Geometry: final body of the model. Coordinates: model frame, mm. Face numbers are marked on the shaded views. A direction names the side the tool comes from. Give positions to 0.01 mm unless a question says otherwise; leave off trailing zeros. Write each loop counter-clockwise with the first axis right and the second up, starting at its lowest first coordinate (ties: lowest second). Pieces come first, ordered by that corner, then holes. Notation, with made-up numbers: (27, 10.5) -> (82, 10.5) arc R18 ccw to (82, 26.5) -> close; hole circle Ø4 at (-2, 69.5). An arc over 180 degrees is marked (long way). Answer as a JSON object with one key per item and string values. Group by question number.
(1) Section query C-C on y = 12. Output: boundary loops of the cut face in (x, z).
(2) Contact query for flat-ended pins moving along their axis: pin 1 Ø4.5 at (x, y) = (6.46, 12) entering from -Z; pin 2 Ø6 at (x, z) = (-3, -2) entering from -Y; pin 3 Ø3 at (x, z) = (-11, -11) entering from +Y. Output: stop coordinate, or through.
(3) Material intervals for probe 1 along X at (y, z) = (1.95, 0); probe 2 along Z at (x, y) = (11, 8.25); probe 3 along Y at (x, z) = (10.5, -2.5), sorted ascending.
(4) Set-up query: the marked faces 1 and 2. Return all of +Z, -Z, +X, -X, +Y, -Y with unobstructed straight access to the full face (end or side cutting, diameter ignored); none if empty.
(5) Section query A-A on x = 0. Output: boundary loops of the cut face in (y, z), plus the area to 3 significant figures.
(6) Section query B-B on z = -6.25. Output: boundary loops of the cut face in (x, y), plus the area to 3 significant figures.
(7) Section query D-D on y = 9.25. Output: boundary loops of the cut face in (x, z), plus the area to 3 significant figures.
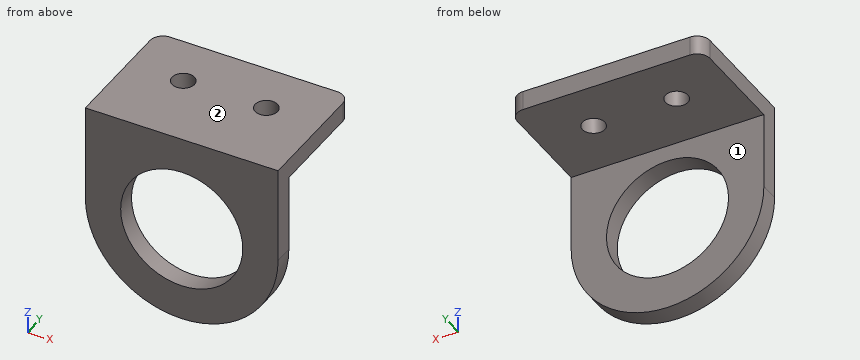
from build123d import *

# Parameters (mm, degrees)
SKETCH_1_R          = 9.5
EXTRUDE_2_DEPTH     = 3
SKETCH_9_W          = 30
SKETCH_9_H          = 20
EXTRUDE_3_DEPTH     = 3
SKETCH_10_R         = 1.75
CUT_EXTRUDE_1_DEPTH = 37.796738986
FILLET_6_R          = 2


with BuildPart() as part:
    # 草图1 → 凸台-拉伸2 (new body)
    with BuildSketch(Plane(origin=(0, 0, 0), x_dir=(1, 0, 0), z_dir=(0, 1, 0))):
        with BuildLine():
            Line((15, -15), (15, 0))
            ThreePointArc((15, 0), (0, 15), (-15, 0))
            Line((-15, 0), (-15, -15))
            Line((-15, -15), (15, -15))
        make_face()
        with Locations(Location((0, 0, 0), (0, 0, 270))):
            Circle(SKETCH_1_R, mode=Mode.SUBTRACT)
    extrude(amount=EXTRUDE_2_DEPTH)

    # 草图9 → 凸台-拉伸3 (add)
    with BuildSketch(Plane.XY.offset(15)):
        with Locations((0, 10)):
            Rectangle(SKETCH_9_W, SKETCH_9_H)
    extrude(amount=-EXTRUDE_3_DEPTH)

    # 草图10 → 切除-拉伸1 (cut, through all)
    with BuildSketch(Plane(origin=(0, 0, 12), x_dir=(-1, 0, 0), z_dir=(0, 0, -1))):
        with Locations((6.461379144, 12)):
            Circle(SKETCH_10_R)
        with Locations(Location((-6.461379144, 12, 0), (0, 0, 180))):
            Circle(SKETCH_10_R)
    extrude(amount=-CUT_EXTRUDE_1_DEPTH, mode=Mode.SUBTRACT)

    # 圆角6
    fillet_6_edges = [part.edges().sort_by_distance(p)[0] for p in [
        (-15, 20, 13.5),
        (15, 20, 13.5),
    ]]
    fillet(fillet_6_edges, radius=FILLET_6_R)


solid = part.part
Answer list:
{
 "1": {"outline": "(-15, 12) -> (-8.21, 12) -> (-8.21, 15) -> (-15, 15) -> close; (-4.71, 12) -> (4.71, 12) -> (4.71, 15) -> (-4.71, 15) -> close; (8.21, 12) -> (15, 12) -> (15, 15) -> (8.21, 15) -> close"},
 "2": {"pin 1": "z = 12", "pin 2": "through", "pin 3": "y = 3"},
 "3": {"probe 1": "-15 to -9.5, 9.5 to 15", "probe 2": "12 to 15", "probe 3": "0 to 3"},
 "4": {"face 1": "-Z, +X, -X, +Y", "face 2": "+Z, +X, -X, +Y, -Y"},
 "5": {"outline": "(0, -15) -> (3, -15) -> (3, -9.5) -> (0, -9.5) -> close; (0, 9.5) -> (3, 9.5) -> (3, 12) -> (20, 12) -> (20, 15) -> (0, 15) -> close", "area": "84.0 mm2"},
 "6": {"outline": "(-13.64, 0) -> (-7.15, 0) -> (-7.15, 3) -> (-13.64, 3) -> close; (7.15, 0) -> (13.64, 0) -> (13.64, 3) -> (7.15, 3) -> close", "area": "38.9 mm2"},
 "7": {"outline": "(-15, 12) -> (15, 12) -> (15, 15) -> (-15, 15) -> close", "area": "90.0 mm2"}
}
